from build123d import *

# Parameters (mm, degrees)
ESBO_O1_R                = 3
RESSALTO_EXTRUS_O1_DEPTH = 360


with BuildPart() as part:
    # Esboço1 → Ressalto-extrusão1 (new body)
    with BuildSketch(Plane.XY):
        Polygon((-2.939339828, 4), (2.939339828, 4), (7.439339828, 8.5), (4, 8.5), (4, 10), (10, 10), (10, 4), (8.5, 4), (8.5, 7.439339828), (4, 2.939339828), (4, -2.939339828), (8.5, -7.439339828), (8.5, -4), (10, -4), (10, -10), (4, -10), (4, -8.5), (7.439339828, -8.5), (2.939339828, -4), (-2.939339828, -4), (-7.439339828, -8.5), (-4, -8.5), (-4, -10), (-10, -10), (-10, -4), (-8.5, -4), (-8.5, -7.439339828), (-4, -2.939339828), (-4, 2.939339828), (-8.5, 7.439339828), (-8.5, 4), (-10, 4), (-10, 10), (-4, 10), (-4, 8.5), (-7.439339828, 8.5), align=None)
        Circle(ESBO_O1_R, mode=Mode.SUBTRACT)
    extrude(amount=RESSALTO_EXTRUS_O1_DEPTH)


solid = part.part
Here's how the part is built. I have some questions about the finished solid (model axes, mm). A direction names the side the tool comes from. Coordinates: 2 decimals unless noted, no trailing zeros. Order: outer loops, then holes, each group sorted by start corner. A loop starts at its lowest first (then second) coordinate and runs counter-clockwise, first axis right, second up.
Item 1: If we section it at A-A on y = 0: List the corners of the cut face in (x, z) for me.
Result sheet:
outline: (-4, 0) - (-3, 0) - (-3, 360) - (-4, 360) - close; (3, 0) - (4, 0) - (4, 360) - (3, 360) - close
Item 2: I need wall thicknesses on line 1 (Y direction, x = 0, z = 317.5); line 2 (Y direction, x = 8.75, z = 264.5); line 3 (X direction, y = -4.5, z = 85.5). Which ranges of each line are inside material? Lowest first, please.
Result sheet:
line 1: y = -4 to -3, 3 to 4
line 2: y = -10 to -4, 4 to 10
line 3: x = -10 to -8.5, -5.56 to -3.44, 3.44 to 5.56, 8.5 to 10
Item 3: For P1, Ø2, axis at y = 1.5, z = 320.5, coming from the -X side; P2, Ø4.5, axis at y = 1, z = 139, coming from the -X side; P3, Ø3, axis at y = 1.5, z = 244, coming from the +X side, each with a flat end and sliding along its axis, tell me the tip position at first contact or that it passes through.
Result sheet:
P1: stops at x = -4
P2: stops at x = -4.31
P3: stops at x = 4.06
Item 4: If we mould it in two halves opening along X, with no side actions, what happens to faces 1 (the face through (7, 10, 177)), 2 (the face through (10, -7, 177)), 3 (the face through (0, 4, 177)), 4 (the face through (0, -4, 177))? For each: +X half, -X half, draft (parallel to the pull), parting line (faces both ways), or undercut.
Result sheet:
face 1: draft
face 2: +X half
face 3: undercut
face 4: undercut
Item 5: For faces 5 (the face through (-3, 0, 177)), 6 (the face through (-4, 0, 177)), 7 (the face through (4, 0, 177)), which set-ups out of +Z, -Z, +X, -X, +Y, -Y let a thin tool reach every point of the face, with its end or its side?
Result sheet:
face 5: +Z, -Z
face 6: +Z, -Z, -X
face 7: +Z, -Z, +X
